```python
from build123d import *

# Parameters (mm, degrees)
SKETCH1_W            = 45.5
SKETCH1_H            = 20.2
BOSS_EXTRUDE1_DEPTH  = 1.6
SKETCH2_R            = 8
BOSS_EXTRUDE2_DEPTH  = 14
SKETCH3_R            = 6.893962295
CUT_EXTRUDE1_DEPTH   = 2
FILLET1_R            = 1
FILLET2_R            = 1
FILLET1_OF_MIRROR1_R = 1
FILLET2_OF_MIRROR1_R = 1
BOSS_EXTRUDE3_DEPTH  = 2
SKETCH5_W            = 0.6
SKETCH5_H            = 0.6
BOSS_EXTRUDE4_DEPTH  = 6
CHAMFER1_SIZE        = 0.1
CHAMFER2_SIZE        = 0.1
CUT_EXTRUDE2_REACH   = 3.6
SKETCH6_R            = 1.05


with BuildPart() as part:
    # Sketch1 → Boss-Extrude1 (new body)
    with BuildSketch(Plane(origin=(0, 0, 0), x_dir=(1, 0, 0), z_dir=(0, 1, 0))):
        with Locations((22.75, 10.1)):
            Rectangle(SKETCH1_W, SKETCH1_H)
    extrude(amount=BOSS_EXTRUDE1_DEPTH)

    # Sketch2 → Boss-Extrude2 (add)
    with BuildSketch(Plane(origin=(0, 1.6, 0), x_dir=(1, 0, 0), z_dir=(0, 1, 0))):
        with Locations((10, 10.1)):
            Circle(SKETCH2_R)
    boss_extrude2 = extrude(amount=BOSS_EXTRUDE2_DEPTH)

    # Sketch3 → Cut-Extrude1 (cut)
    with BuildSketch(Plane(origin=(0, 15.6, 0), x_dir=(1, 0, 0), z_dir=(0, 1, 0))):
        with Locations((10, 10.1)):
            Circle(SKETCH3_R)
    cut_extrude1 = extrude(amount=-CUT_EXTRUDE1_DEPTH, mode=Mode.SUBTRACT)

    # Fillet1
    fillet1_edges = [part.edges().sort_by_distance(p)[0] for p in [
        (2, 15.6, -10.1),
    ]]
    fillet(fillet1_edges, radius=FILLET1_R)

    # Fillet2
    fillet2_edges = [part.edges().sort_by_distance(p)[0] for p in [
        (3.106037705, 13.6, -10.1),
    ]]
    fillet(fillet2_edges, radius=FILLET2_R)

    # Mirror1: Boss-Extrude2, Cut-Extrude1 across plane
    add(boss_extrude2.mirror(Plane(origin=(22.75, 0, 0), x_dir=(0, 0, 1), z_dir=(1, 0, 0))))
    add(cut_extrude1.mirror(Plane(origin=(22.75, 0, 0), x_dir=(0, 0, 1), z_dir=(1, 0, 0))), mode=Mode.SUBTRACT)

    # Fillet1 of Mirror1
    fillet1_of_mirror1_edges = [part.edges().sort_by_distance(p)[0] for p in [
        (43.5, 15.6, -10.1),
    ]]
    fillet(fillet1_of_mirror1_edges, radius=FILLET1_OF_MIRROR1_R)

    # Fillet2 of Mirror1
    fillet2_of_mirror1_edges = [part.edges().sort_by_distance(p)[0] for p in [
        (42.393962295, 13.6, -10.1),
    ]]
    fillet(fillet2_of_mirror1_edges, radius=FILLET2_OF_MIRROR1_R)

    # Sketch4 → Boss-Extrude3 (add)
    with BuildSketch(Plane(origin=(0, 1.6, 0), x_dir=(1, 0, 0), z_dir=(0, 1, 0))):
        Polygon((22.75, 0), (19.9, 0), (19.9, 2.7), (25.6, 2.7), (25.6, 0), align=None)
    extrude(amount=BOSS_EXTRUDE3_DEPTH)

    # Sketch5 → Boss-Extrude4 (add)
    with BuildSketch(Plane.XY):
        with Locations((20.606248373, 2.6)):
            Rectangle(SKETCH5_W, SKETCH5_H)
        with Locations((22.036248373, 2.6)):
            Rectangle(SKETCH5_W, SKETCH5_H)
        with Locations((23.466248373, 2.6)):
            Rectangle(SKETCH5_W, SKETCH5_H)
        with Locations((24.896248373, 2.6)):
            Rectangle(SKETCH5_W, SKETCH5_H)
    extrude(amount=BOSS_EXTRUDE4_DEPTH)

    # Chamfer1
    chamfer1_edges = [part.edges().sort_by_distance(p)[0] for p in [
        (20.906248373, 2.3, 3),
        (20.906248373, 2.9, 3),
        (20.306248373, 2.9, 3),
        (20.306248373, 2.3, 3),
        (20.906248373, 2.6, 6),
        (20.606248373, 2.9, 6),
        (20.306248373, 2.6, 6),
        (20.606248373, 2.3, 6),
        (22.336248373, 2.9, 3),
        (21.736248373, 2.9, 3),
        (21.736248373, 2.3, 3),
        (22.336248373, 2.3, 3),
        (22.036248373, 2.9, 6),
        (21.736248373, 2.6, 6),
        (22.036248373, 2.3, 6),
        (22.336248373, 2.6, 6),
        (23.766248373, 2.9, 3),
        (23.166248373, 2.9, 3),
        (23.166248373, 2.3, 3),
        (23.766248373, 2.3, 3),
        (23.466248373, 2.9, 6),
        (23.166248373, 2.6, 6),
        (23.466248373, 2.3, 6),
        (23.766248373, 2.6, 6),
        (25.196248373, 2.9, 3),
        (24.596248373, 2.9, 3),
        (24.596248373, 2.3, 3),
        (25.196248373, 2.3, 3),
        (24.896248373, 2.9, 6),
        (24.596248373, 2.6, 6),
        (24.896248373, 2.3, 6),
        (25.196248373, 2.6, 6),
    ]]
    chamfer(chamfer1_edges, length=CHAMFER1_SIZE)

    # Chamfer2
    chamfer2_edges = [part.edges().sort_by_distance(p)[0] for p in [
        (22.75, 3.6, 0),
        (25.6, 3.6, -1.35),
        (22.75, 3.6, -2.7),
        (19.9, 3.6, -1.35),
    ]]
    chamfer(chamfer2_edges, length=CHAMFER2_SIZE)

    # Sketch6 → Cut-Extrude2 (cut, up to next)
    with BuildSketch(Plane(origin=(0, 1.6, 0), x_dir=(1, 0, 0), z_dir=(0, 1, 0)), mode=Mode.PRIVATE) as cut_extrude2_sk1:
        with Locations((1.7, 18.5)):
            Circle(SKETCH6_R)
    cut_extrude2_tool1 = extrude(cut_extrude2_sk1.sketch, amount=-CUT_EXTRUDE2_REACH, mode=Mode.PRIVATE) & part.part
    add(cut_extrude2_tool1.solids().sort_by_distance((1.7, 1.6, -18.5))[0], mode=Mode.SUBTRACT)
    # Sketch6 → Cut-Extrude2 (cut, up to next)
    with BuildSketch(Plane(origin=(0, 1.6, 0), x_dir=(1, 0, 0), z_dir=(0, 1, 0)), mode=Mode.PRIVATE) as cut_extrude2_sk2:
        with Locations((1.7, 1.7)):
            Circle(SKETCH6_R)
    cut_extrude2_tool2 = extrude(cut_extrude2_sk2.sketch, amount=-CUT_EXTRUDE2_REACH, mode=Mode.PRIVATE) & part.part
    add(cut_extrude2_tool2.solids().sort_by_distance((1.7, 1.6, -1.7))[0], mode=Mode.SUBTRACT)
    # Sketch6 → Cut-Extrude2 (cut, up to next)
    with BuildSketch(Plane(origin=(0, 1.6, 0), x_dir=(1, 0, 0), z_dir=(0, 1, 0)), mode=Mode.PRIVATE) as cut_extrude2_sk3:
        with Locations((43.8, 1.7)):
            Circle(SKETCH6_R)
    cut_extrude2_tool3 = extrude(cut_extrude2_sk3.sketch, amount=-CUT_EXTRUDE2_REACH, mode=Mode.PRIVATE) & part.part
    add(cut_extrude2_tool3.solids().sort_by_distance((43.8, 1.6, -1.7))[0], mode=Mode.SUBTRACT)
    # Sketch6 → Cut-Extrude2 (cut, up to next)
    with BuildSketch(Plane(origin=(0, 1.6, 0), x_dir=(1, 0, 0), z_dir=(0, 1, 0)), mode=Mode.PRIVATE) as cut_extrude2_sk4:
        with Locations((43.8, 18.5)):
            Circle(SKETCH6_R)
    cut_extrude2_tool4 = extrude(cut_extrude2_sk4.sketch, amount=-CUT_EXTRUDE2_REACH, mode=Mode.PRIVATE) & part.part
    add(cut_extrude2_tool4.solids().sort_by_distance((43.8, 1.6, -18.5))[0], mode=Mode.SUBTRACT)


solid = part.part
```
Check sheet for the modelled part. Datum: model origin and axes. Units: mm. A direction names the side the tool comes from. Round coordinates to 2 decimals unless told otherwise and drop trailing zeros. Order: outer loops, then holes, each group sorted by start corner. A loop starts at its lowest first (then second) coordinate and runs counter-clockwise, first axis right, second up. Notation, with made-up numbers: (62.25, -32.5) - (81.25, -32.5) arc R29 ccw to (81.25, -11.5) - close; hole circle Ø11 at (-30.5, 79). An arc over 180 degrees is marked (long way). Write item = value, one per line.
Q1. Go/stop test with flat-tipped pins: pin 1 (11 mm diameter, centred on x = 10, z = -10.1, fed in from +Y); pin 2 (1 mm diameter, centred on y = 2.5, z = -1.5, fed in from -X); pin 3 (4 mm diameter, centred on x = 20, z = -17, fed in from +Y); pin 4 (1.7 mm diameter, centred on x = 1.7, z = -1.7, fed in from -Y). Record where each tip stops, or that it passes through.
Computed:
pin_1 = 13.6
pin_2 = 19.9
pin_3 = 1.6
pin_4 = through
Q2. Section check A-A (z = 1.25). State how many separate pieces and enclosed holes the cut face has, and give its area (3 significant figures).
Computed:
separate_pieces = 4
enclosed_holes = 0
area = 1.36 mm^2
Q3. Section check C-C (z = -10.1). Record the boundary of the cut face in (x, y), and give its area (3 significant figures).
Computed:
outline = (0, 0) - (45.5, 0) - (45.5, 1.6) - (43.5, 1.6) - (43.5, 14.6) arc R1 ccw to (42.5, 15.6) - (42.39, 15.6) - (42.39, 14.6) arc R1 cw to (41.39, 13.6) - (29.61, 13.6) arc R1 cw to (28.61, 14.6) - (28.61, 15.6) - (28.5, 15.6) arc R1 ccw to (27.5, 14.6) - (27.5, 1.6) - (18, 1.6) - (18, 14.6) arc R1 ccw to (17, 15.6) - (16.89, 15.6) - (16.89, 14.6) arc R1 cw to (15.89, 13.6) - (4.11, 13.6) arc R1 cw to (3.11, 14.6) - (3.11, 15.6) - (3, 15.6) arc R1 ccw to (2, 14.6) - (2, 1.6) - (0, 1.6) - close
area = 466 mm^2
Q4. Draft check along X on faces 4 (the face through (45.5, 1, -10)), 5 (the face through (8.27, 8.01, -2.29)), 6 (the face through (44.77, 0.81, -1.3)), 7 (the face through (0, 1, -10)). Enter one of: pulls with the +X half, pulls with the -X half, needs draft (parallel to the pull), parting line crosses it, or undercut.
Computed:
face_4 = pulls with the +X half
face_5 = undercut
face_6 = undercut
face_7 = pulls with the -X half
Q5. Section check B-B (x = 10). Record the boundary of the cut face in (y, z).
Computed:
outline = (0, -20.2) - (1.6, -20.2) - (1.6, -18.1) - (14.6, -18.1) arc R1 ccw to (15.6, -17.1) - (15.6, -16.99) - (14.6, -16.99) arc R1 cw to (13.6, -15.99) - (13.6, -4.21) arc R1 cw to (14.6, -3.21) - (15.6, -3.21) - (15.6, -3.1) arc R1 ccw to (14.6, -2.1) - (1.6, -2.1) - (1.6, 0) - (0, 0) - close
Q6. Thickness scan on line 1 along X through (y, z) = (1.15, -18.5); line 2 along X through (y, z) = (15.4, -10.1); line 3 along X through (y, z) = (14.9, -10.1). Record the ranges inside material, lowest first.
Computed:
line_1 = 0 to 0.65, 2.75 to 42.75, 44.85 to 45.5
line_2 = 2.4 to 3.11, 16.89 to 17.6, 27.9 to 28.61, 42.39 to 43.1
line_3 = 2.05 to 3.11, 16.89 to 17.95, 27.55 to 28.61, 42.39 to 43.45
Q7. Section check D-D (y = 8). Record the boundary of the cut face in (x, z).
Computed:
outline = circle Ø16 at (10, -10.1); circle Ø16 at (35.5, -10.1)
Q8. Tool access check on faces 1 (the face through (10, 13.6, -10)), 2 (the face through (19.9, 3, -1)), 3 (the face through (23, 3, -2.7)). Record the directions out of +Z, -Z, +X, -X, +Y, -Y that give a thin tool (end or side, any length) a straight path to the whole face; none if there is none.
Computed:
face_1 = +Y
face_2 = +Z, -Z, +Y
face_3 = -Z, +Y
